```python
from build123d import *

# Parameters (mm, degrees)
CHAMFER1_SIZE = 0.1984375
FILLET1_R     = 0.1984375
FILLET2_R     = 0.09921875


with BuildPart() as part:
    # Sketch3 → Revolve1 (revolve)
    with BuildSketch(Plane(origin=(0, 0, 0), x_dir=(0, 0, -1), z_dir=(1, 0, 0))):
        Polygon((3.175, 6.35), (1.5875, 6.35), (1.5875, 4.7752), (-3.175, 4.7752), (-3.175, 3.1877), (3.175, 3.1877), align=None)
    revolve(axis=Axis((0, 0, -3.175), (0, 0, 1)))

    # Chamfer1
    chamfer1_edges = [part.edges().sort_by_distance(p)[0] for p in [
        (0, -3.1877, 3.175),
        (0, -4.7752, 3.175),
        (0, -6.35, -1.5875),
    ]]
    chamfer(chamfer1_edges, length=CHAMFER1_SIZE)

    # Fillet1
    fillet1_edges = [part.edges().sort_by_distance(p)[0] for p in [
        (0, -6.35, -3.175),
    ]]
    fillet(fillet1_edges, radius=FILLET1_R)

    # Fillet2
    fillet2_edges = [part.edges().sort_by_distance(p)[0] for p in [
        (0, -4.7752, -1.5875),
    ]]
    fillet(fillet2_edges, radius=FILLET2_R)


solid = part.part
```
Work out the finished part from the listing and answer in its coordinate system (mm). A direction names the side the tool comes from. Give positions to 0.01 mm unless a question says otherwise; leave off trailing zeros. Order: outer loops, then holes, each group sorted by start corner. A loop starts at its lowest first (then second) coordinate and runs counter-clockwise, first axis right, second up.
1. Section D-D, the plane z = 2.5 is taken. Determine the outline of the cut face in (x, y).
Result sheet:
outline: circle Ø9.55 at (0, 0); hole circle Ø6.38 at (0, 0)
2. Straight lines are drawn through the part: L1, parallel to X at y = 0, z = -0.75; L2, parallel to Z at x = -5, y = 2 (1 decimal). For each, find the intervals that lie inside material, in ascending order.
Result sheet:
L1: x = -4.78 to -3.19, 3.19 to 4.78
L2: z = -3.2 to -1.6
3. Section C-C, the plane z = -2.5 is taken. Determine the outline of the cut face in (x, y), and give its area (3 significant figures).
Result sheet:
outline: circle Ø12.7 at (0, 0); hole circle Ø6.38 at (0, 0)
area: 94.8 mm2
4. The mould has two halves that part along Y. Classify faces 1 (the flat face through (3, -3, -3.175)), 2 (the cylindrical face through (2.83, 1.47, -0.14)), 3 (the cylindrical face through (6.2, -1.38, -2.37)): released by +Y, released by -Y, zero draft, split by the parting line, or undercut.
Result sheet:
face 1: zero draft
face 2: undercut
face 3: split by the parting line
5. Each of these flat-tipped pins is pushed along its axis until it touches: P1, Ø1.5, axis at x = -1.5, z = -2.5, coming from the -Y side; P2, Ø1, axis at y = -3, z = -1, coming from the -X side; P3, Ø2, axis at y = 1.5, z = -2, coming from the -X side. Where does it stop, or does it pass through?
Result sheet:
P1: stops at y = -6.31
P2: stops at x = -4.07
P3: stops at x = -6.33
6. For faces 4 (the flat face through (-5, -2, -1.588)), 5 (the flat face through (2, -3, 3.175)), determine the directions among +Z, -Z, +X, -X, +Y, -Y from which every point of the face is accessible in a straight line to the end or side of a thin tool.
Result sheet:
face 4: +Z
face 5: +Z, +X, -X, +Y, -Y
